Source: CAD feature listing. Evaluate the final solid. Frame: model axes, mm. Round coordinates to 2 decimals unless told otherwise and drop trailing zeros. Loops run counter-clockwise (first coordinate to the right, second up) from the corner with the lowest first, then second, coordinate; pieces in that order, holes last. Notation, with made-up numbers: (7.5, 68.5) - (60.5, 68.5) arc R23 cw to (60.5, 106.5) - close; hole circle Ø9 at (72.5, -33). An arc over 180 degrees is marked (long way). One line per question, with ' | ' between items.
from build123d import *

# Parameters (mm, degrees)
SKETCH1_W                 = 267.22
SKETCH1_H                 = 361.68
SKETCH1_R                 = 3.57
SKETCH1_R_2               = 3.7
BOSS_EXTRUDE1_DEPTH       = 10
SKETCH2_W                 = 101.6
SKETCH2_H                 = 101.6
CUT_EXTRUDE1_DEPTH        = 226.066074076
LPATTERN1_COUNT           = 2
LPATTERN1_PITCH           = 110.265
LPATTERN2_COUNT           = 2
LPATTERN2_PITCH           = 110.265
LPATTERN3_COUNT           = 2
LPATTERN3_PITCH           = 114.82
LPATTERN3_COPY_1_SKETCH_W = 101.6
LPATTERN3_COPY_1_SKETCH_H = 101.6
LPATTERN3_COPY_1_DEPTH    = 226.066074076
LPATTERN3_COPY_2_SKETCH_W = 101.6
LPATTERN3_COPY_2_SKETCH_H = 101.6
LPATTERN3_COPY_2_DEPTH    = 226.066074076


with BuildPart() as part:
    # Sketch1 → Boss-Extrude1 (new body)
    with BuildSketch(Plane(origin=(0, 0, 0), x_dir=(1, 0, 0), z_dir=(0, 1, 0))):
        Rectangle(SKETCH1_W, SKETCH1_H)
        with Locations(Location((-120.91, -169.7275, 0), (0, 0, 270))):
            Circle(SKETCH1_R, mode=Mode.SUBTRACT)
        with Locations(Location((-120.91, 169.7275, 0), (0, 0, 270))):
            Circle(SKETCH1_R, mode=Mode.SUBTRACT)
        with Locations(Location((70.11, 169.7275, 0), (0, 0, 270))):
            Circle(SKETCH1_R, mode=Mode.SUBTRACT)
        with Locations(Location((70.11, -169.7275, 0), (0, 0, 270))):
            Circle(SKETCH1_R, mode=Mode.SUBTRACT)
        with Locations(Location((-95.51, 169.7275, 0), (0, 0, 270))):
            Circle(SKETCH1_R, mode=Mode.SUBTRACT)
        with Locations(Location((-95.51, -169.7275, 0), (0, 0, 270))):
            Circle(SKETCH1_R_2, mode=Mode.SUBTRACT)
        with Locations(Location((95.51, 169.7275, 0), (0, 0, 270))):
            Circle(SKETCH1_R, mode=Mode.SUBTRACT)
        with Locations(Location((95.51, -169.7275, 0), (0, 0, 270))):
            Circle(SKETCH1_R, mode=Mode.SUBTRACT)
    extrude(amount=BOSS_EXTRUDE1_DEPTH)

    # Sketch2 → Cut-Extrude1 (cut, through all)
    with BuildSketch(Plane(origin=(0, 10, 0), x_dir=(1, 0, 0), z_dir=(0, 1, 0))):
        with Locations((-70.11, 0)):
            Rectangle(SKETCH2_W, SKETCH2_H)
    cut_extrude1 = extrude(amount=-CUT_EXTRUDE1_DEPTH, mode=Mode.SUBTRACT)

    # LPattern1: Cut-Extrude1 ×2
    with Locations(*[(0, 0, -i * LPATTERN1_PITCH) for i in range(1, LPATTERN1_COUNT)]):
        add(cut_extrude1, mode=Mode.SUBTRACT)

    # LPattern2: Cut-Extrude1 ×2
    with Locations(*[(0, 0, i * LPATTERN2_PITCH) for i in range(1, LPATTERN2_COUNT)]):
        add(cut_extrude1, mode=Mode.SUBTRACT)

    # LPattern3: Cut-Extrude1 ×2
    with Locations(*[(i * LPATTERN3_PITCH, 0, 0) for i in range(1, LPATTERN3_COUNT)]):
        add(cut_extrude1, mode=Mode.SUBTRACT)

    # LPattern3 copy 1 sketch → LPattern3 copy 1 (cut, through all)
    with BuildSketch(Plane(origin=(114.82, 10, -110.265), x_dir=(1, 0, 0), z_dir=(0, 1, 0))):
        with Locations((-70.11, 0)):
            Rectangle(LPATTERN3_COPY_1_SKETCH_W, LPATTERN3_COPY_1_SKETCH_H)
    extrude(amount=-LPATTERN3_COPY_1_DEPTH, mode=Mode.SUBTRACT)

    # LPattern3 copy 2 sketch → LPattern3 copy 2 (cut, through all)
    with BuildSketch(Plane(origin=(114.82, 10, 110.265), x_dir=(1, 0, 0), z_dir=(0, 1, 0))):
        with Locations((-70.11, 0)):
            Rectangle(LPATTERN3_COPY_2_SKETCH_W, LPATTERN3_COPY_2_SKETCH_H)
    extrude(amount=-LPATTERN3_COPY_2_DEPTH, mode=Mode.SUBTRACT)


solid = part.part
1. Mould query, pull axis Z, two halves, no side actions, for faces 1 (the cylindrical face through (96.582, 4.93, 173.133)), 2 (the flat face through (-133.61, 5, 3)). Classes: released by +Z, released by -Z, zero draft, split by the parting line, or undercut.
Worked out:
face 1: undercut | face 2: zero draft
2. Section query B-B, the plane x = -26. Return loops of the section in (y, z) (3 decimals), plus the area to 3 significant figures.
Worked out:
outline: (0, -180.84) - (10, -180.84) - (10, -161.065) - (0, -161.065) - close; (0, -59.465) - (10, -59.465) - (10, -50.8) - (0, -50.8) - close; (0, 50.8) - (10, 50.8) - (10, 59.465) - (0, 59.465) - close; (0, 161.065) - (10, 161.065) - (10, 180.84) - (0, 180.84) - close | area: 569 mm2
3. Contact query for a flat-ended pin moving along its axis: P1, Ø10, axis at x = 17, z = 46, coming from the -Y side. Output: stop coordinate, or through.
Worked out:
P1: stops at y = 0
4. Material intervals for probe 1 along X at (y, z) = (4.25, -129); probe 2 along Z at (x, y) = (-47.5, 5.25) (3 decimals); probe 3 along Z at (x, y) = (72.5, 8) (3 decimals), sorted ascending.
Worked out:
probe 1: x = -133.61 to -120.91, -19.31 to -6.09, 95.51 to 133.61 | probe 2: z = -180.84 to -161.065, -59.465 to -50.8, 50.8 to 59.465, 161.065 to 180.84 | probe 3: z = -180.84 to -172.379, -167.076 to -161.065, -59.465 to -50.8, 50.8 to 59.465, 161.065 to 167.076, 172.379 to 180.84
5. Section query C-C, the plane y = 4.25. Give the number of separate pieces and of enclosed holes in the cut face, plus the area to 3 significant figures.
Worked out:
separate pieces: 1 | enclosed holes: 14 | area: 34,400 mm2
6. Section query A-A, the plane z = 35. Return loops of the section in (x, y), plus the area to 3 significant figures.
Worked out:
outline: (-133.61, 0) - (-120.91, 0) - (-120.91, 10) - (-133.61, 10) - close; (-19.31, 0) - (-6.09, 0) - (-6.09, 10) - (-19.31, 10) - close; (95.51, 0) - (133.61, 0) - (133.61, 10) - (95.51, 10) - close | area: 640 mm2
